For this review, take the finished solid that the model builds, in its own axes (mm). Face numbers are marked on the shaded views. A direction names the side the tool comes from. Give positions to 0.01 mm unless a question says otherwise; leave off trailing zeros. Order: outer loops, then holes, each group sorted by start corner. A loop starts at its lowest first (then second) coordinate and runs counter-clockwise, first axis right, second up.
Item 1: Consider section D-D (x = 2.25). Give the boundary of the cut face in (y, z).
Item 2: Consider section A-A (x = 5.9). Give the boundary of the cut face in (y, z), plus the area to 3 significant figures.
Item 3: For P1, Ø1, axis at x = 2.5, y = 3, coming from the +Z side; P2, Ø1, axis at y = 3, z = -2.5, coming from the -X side; P3, Ø1, axis at x = 1, z = -2, coming from the +Y side, all flat-tipped, find the tip position at first contact; note any pin that passes through.
Item 4: For probe 1 along X at (y, z) = (0.35, -0.55); probe 2 along Y at (x, z) = (0.5, -3); probe 3 along Z at (x, y) = (2.5, 0.85), list the stretches that pass through material, from the lowest coordinate up.
Item 5: The part is to be moulded in two halves that separate along Y. For the marked faces 1, 2 and 3, say which applies: released by +Y, released by -Y, zero draft, split by the parting line, or undercut.
Item 6: Machinability: for the marked faces 4, 5, 6, 7 and 8, which of the approach directions +Z, -Z, +X, -X, +Y, -Y give a long, thin tool a straight path to every point of the face, cutting with its end or side? Answer none if there is none.
Item 7: Consider section B-B (z = -4.25). Give the boundary of the cut face in (x, y).
```python
from build123d import *

# Parameters (mm, degrees)
SKETCH1_R            = 0.15
BOSS_EXTRUDE1_DEPTH  = 0.5
FILLET1_R            = 0.4
FILLET2_R            = 0.16
BOSS_EXTRUDE2_DEPTH  = 1.6
SKETCH3_R            = 0.75
BOSS_EXTRUDE7_DEPTH  = 2
SKETCH4_W            = 1.8
SKETCH4_H            = 1.8
BOSS_EXTRUDE8_DEPTH  = 0.3
SKETCH5_R            = 1.15
BOSS_EXTRUDE9_DEPTH  = 0.7
SKETCH6_W            = 0.9
SKETCH6_H            = 0.3
BOSS_EXTRUDE10_DEPTH = 2
FILLET3_R            = 0.3
SKETCH7_W            = 4.7
SKETCH7_H            = 0.3
BOSS_EXTRUDE11_DEPTH = 0.01


with BuildPart() as part:
    # Sketch1 → Boss-Extrude1 (new body)
    with BuildSketch(Plane(origin=(0, 0, 0), x_dir=(1, 0, 0), z_dir=(0, 1, 0))):
        Polygon((0, 0), (1.1, 0), (1.1, 0.7), (5.4, 0.7), (5.4, 0), (6.4, 0), (6.4, 0.7), (6.2, 0.7), (6.2, 4.1), (6.4, 4.1), (6.4, 4.9), (5.4, 4.9), (5.4, 4.1), (1.1, 4.1), (1.1, 4.9), (0, 4.9), (0, 4.1), (0.2, 4.1), (0.2, 0.7), (0, 0.7), align=None)
        with Locations(Location((0.5, 4.25, 0), (0, 0, 270))):
            Circle(SKETCH1_R, mode=Mode.SUBTRACT)
        with Locations(Location((0.5, 0.55, 0), (0, 0, 270))):
            Circle(SKETCH1_R, mode=Mode.SUBTRACT)
        with Locations(Location((5.9, 0.55, 0), (0, 0, 270))):
            Circle(SKETCH1_R, mode=Mode.SUBTRACT)
        with Locations(Location((5.9, 4.25, 0), (0, 0, 270))):
            Circle(SKETCH1_R, mode=Mode.SUBTRACT)
    extrude(amount=BOSS_EXTRUDE1_DEPTH)

    # Fillet1
    fillet1_edges = [part.edges().sort_by_distance(p)[0] for p in [
        (1.1, 0.25, -4.1),
        (5.4, 0.25, -4.1),
        (5.4, 0.25, -0.7),
        (1.1, 0.25, -0.7),
    ]]
    fillet(fillet1_edges, radius=FILLET1_R)

    # Fillet2
    fillet2_edges = [part.edges().sort_by_distance(p)[0] for p in [
        (0, 0.25, -0.7),
        (0.2, 0.25, -4.1),
        (0, 0.25, -4.9),
        (6.4, 0.25, -4.9),
        (6.2, 0.25, -4.1),
        (6.2, 0.25, -0.7),
        (6.4, 0.25, 0),
        (0, 0.25, 0),
    ]]
    fillet(fillet2_edges, radius=FILLET2_R)

    # Sketch2 → Boss-Extrude2 (add)
    with BuildSketch(Plane(origin=(0, 0.5, 0), x_dir=(1, 0, 0), z_dir=(0, 1, 0))):
        Polygon((0.2, 0.83), (5.5, 0.83), (5.5, 2.4), (3, 2.4), (3, 3.97), (0.2, 3.97), align=None)
    extrude(amount=BOSS_EXTRUDE2_DEPTH)

    # Sketch3 → Boss-Extrude7 (add)
    with BuildSketch(Plane(origin=(3, 0, 0), x_dir=(0, 0, -1), z_dir=(1, 0, 0))):
        with Locations(Location((3.185, 1.3, 0), (0, 0, 180))):
            Circle(SKETCH3_R)
    extrude(amount=BOSS_EXTRUDE7_DEPTH)

    # Sketch4 → Boss-Extrude8 (add)
    with BuildSketch(Plane.XZ):
        with Locations((3.25, -2.32)):
            Rectangle(SKETCH4_W, SKETCH4_H)
    extrude(amount=BOSS_EXTRUDE8_DEPTH)

    # Sketch5 → Boss-Extrude9 (add)
    with BuildSketch(Plane.ZY.offset(-0.2)):
        with Locations(Location((-1.575, 1.05, 0), (0, 0, 114.070614623))):
            Circle(SKETCH5_R)
    extrude(amount=BOSS_EXTRUDE9_DEPTH)

    # Sketch6 → Boss-Extrude10 (add)
    with BuildSketch(Plane(origin=(0, 2.1, 0), x_dir=(1, 0, 0), z_dir=(0, 1, 0))):
        with Locations((2.497976847, 1.617210326)):
            Rectangle(SKETCH6_W, SKETCH6_H)
    extrude(amount=BOSS_EXTRUDE10_DEPTH)

    # Fillet3
    fillet3_edges = [part.edges().sort_by_distance(p)[0] for p in [
        (2.047976847, 4.1, -1.617210326),
        (2.947976847, 4.1, -1.617210326),
    ]]
    fillet(fillet3_edges, radius=FILLET3_R)

    # Sketch7 → Boss-Extrude11 (add)
    with BuildSketch(Plane(origin=(0, 2.1, 0), x_dir=(1, 0, 0), z_dir=(0, 1, 0))):
        with Locations((2.85, 1.617210326)):
            Rectangle(SKETCH7_W, SKETCH7_H)
    extrude(amount=BOSS_EXTRUDE11_DEPTH)


solid = part.part
```
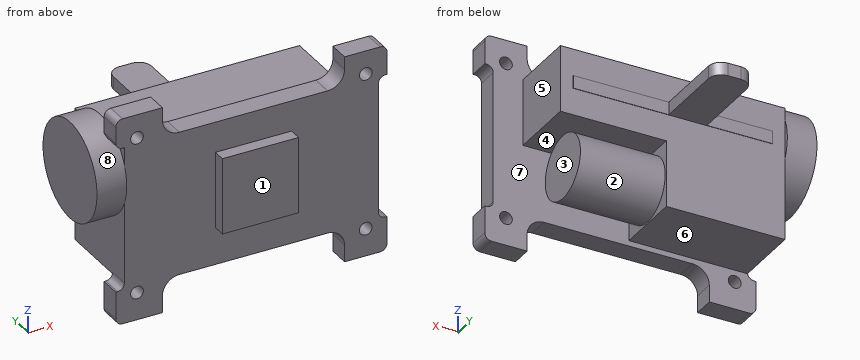
Resolved:
1. outline: (0, -4.1) - (0.5, -4.1) - (0.5, -3.97) - (2.1, -3.97) - (2.1, -1.77) - (4.08, -1.77) - (4.08, -1.47) - (2.1, -1.47) - (2.1, -0.83) - (0.5, -0.83) - (0.5, -0.7) - (0, -0.7) - close
2. outline: (0, -4.9) - (0.5, -4.9) - (0.5, -4.4) - (0, -4.4) - close; (0, -4.1) - (0.5, -4.1) - (0.5, -0.7) - (0, -0.7) - close; (0, -0.4) - (0.5, -0.4) - (0.5, 0) - (0, 0) - close
2. area: 2.15 mm2
3. P1: stops at z = -1.47
3. P2: passes through
3. P3: stops at y = 2.11
4. probe 1: x = 0 to 0.35, 0.65 to 1.19, 5.31 to 5.75, 6.05 to 6.4
4. probe 2: y = 0 to 2.1
4. probe 3: z = -3.97 to -0.83
5. face 1: released by -Y
5. face 2: undercut
5. face 3: zero draft
6. face 4: +X, +Y
6. face 5: +Z, -Z, +X, +Y
6. face 6: -Z, +X, -X, +Y
6. face 7: +X
6. face 8: -X
7. outline: (0, 0) - (0.35, 0) - (0.35, 0.5) - (0, 0.5) - close; (0.65, 0) - (1.19, 0) - (1.19, 0.5) - (0.65, 0.5) - close; (5.31, 0) - (5.75, 0) - (5.75, 0.5) - (5.31, 0.5) - close; (6.05, 0) - (6.4, 0) - (6.4, 0.5) - (6.05, 0.5) - close
